Here's how the part is built. I have some questions about the finished solid (model axes, mm). Give positions to 0.01 mm unless a question says otherwise; leave off trailing zeros. Order: outer loops, then holes, each group sorted by start corner. A loop starts at its lowest first (then second) coordinate and runs counter-clockwise, first axis right, second up.
from build123d import *

# Parameters (mm, degrees)
SKETCH_1_W          = 61.702142611
SKETCH_1_H          = 61.347239899
EXTRUDE_1_DEPTH     = 2
SKETCH_2_W          = 9
SKETCH_2_H          = 6
CUT_EXTRUDE_1_DEPTH = 2


with BuildPart() as part:
    # 草图1 → 凸台-拉伸1 (new body)
    with BuildSketch(Plane(origin=(-129.641159043, -2421.788142989, -243.940490516), x_dir=(1, 0, 0), z_dir=(0, 1, 0))):
        with BuildLine():
            Line((-116.231072015, -154.924864972), (-44.528929404, -154.924864972))
            ThreePointArc((-44.528929404, -154.924864972), (-43.114715842, -155.510651409), (-42.528929404, -156.924864972))
            Line((-42.528929404, -156.924864972), (-42.528929404, -226.272104871))
            ThreePointArc((-42.528929404, -226.272104871), (-43.114715842, -227.686318433), (-44.528929404, -228.272104871))
            Line((-44.528929404, -228.272104871), (-116.231072015, -228.272104871))
            ThreePointArc((-116.231072015, -228.272104871), (-117.645285578, -227.686318433), (-118.231072015, -226.272104871))
            Line((-118.231072015, -226.272104871), (-118.231072015, -156.924864972))
            ThreePointArc((-118.231072015, -156.924864972), (-117.645285578, -155.510651409), (-116.231072015, -154.924864972))
        make_face()
        with Locations((-80.38000071, -191.598484922)):
            Rectangle(SKETCH_1_W, SKETCH_1_H, mode=Mode.SUBTRACT)
    extrude(amount=EXTRUDE_1_DEPTH)

    # 草图2 → 切除-拉伸1 (cut)
    with BuildSketch(Plane(origin=(0, -2419.788142989, 0), x_dir=(1, 0, 0), z_dir=(0, 1, 0))):
        with Locations((-232.033164197, 86.015625544)):
            Rectangle(SKETCH_2_W, SKETCH_2_H)
    extrude(amount=-CUT_EXTRUDE_1_DEPTH, mode=Mode.SUBTRACT)


solid = part.part
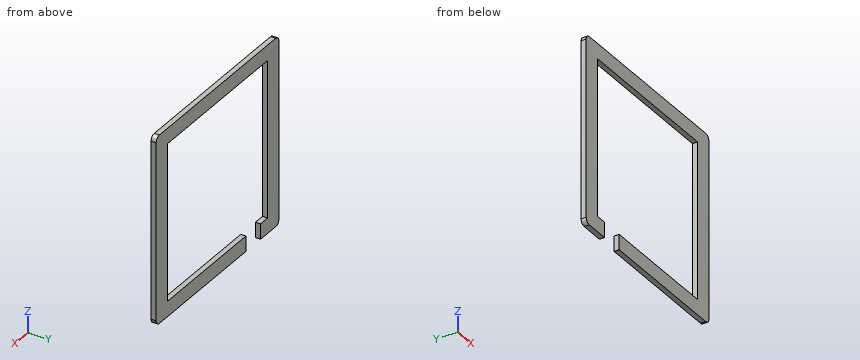
Q1. I'm going to push a flat-ended pin straight in: P1, Ø10, axis at x = -206, z = -80, coming from the +Y side. Where does the tip first touch, or does it pass through?
Filled sheet:
P1: stops at y = -2419.79
Q2. If we section it at C-C on y = -2421.25: List the corners of the cut face in (x, z) for me, plus the area to 3 significant figures.
Filled sheet:
outline: (-247.87, -87.02) arc R2 ccw to (-245.87, -89.02) - (-236.53, -89.02) - (-236.53, -83.02) - (-240.87, -83.02) - (-240.87, -21.67) - (-179.17, -21.67) - (-179.17, -83.02) - (-227.53, -83.02) - (-227.53, -89.02) - (-174.17, -89.02) arc R2 ccw to (-172.17, -87.02) - (-172.17, -17.67) arc R2 ccw to (-174.17, -15.67) - (-245.87, -15.67) arc R2 ccw to (-247.87, -17.67) - close
area: 1,710 mm2
Q3. I need wall thicknesses on L1, parallel to X at y = -2421.05, z = -73; L2, parallel to Z at x = -196.5, y = -2421.5; L3, parallel to Z at x = -236, y = -2420.5. Which ranges of each line are inside material? Lowest first, please.
Filled sheet:
L1: x = -247.87 to -240.87, -179.17 to -172.17
L2: z = -89.02 to -83.02, -21.67 to -15.67
L3: z = -21.67 to -15.67
Q4. If we section it at A-A on x = -189.5: List the corners of the cut face in (y, z) for me.
Filled sheet:
outline: (-2421.79, -89.02) - (-2419.79, -89.02) - (-2419.79, -83.02) - (-2421.79, -83.02) - close; (-2421.79, -21.67) - (-2419.79, -21.67) - (-2419.79, -15.67) - (-2421.79, -15.67) - close
Q5. If we section it at D-D on x = -229.5: List the corners of the cut face in (y, z) for me.
Filled sheet:
outline: (-2421.79, -21.67) - (-2419.79, -21.67) - (-2419.79, -15.67) - (-2421.79, -15.67) - close
Q6. If we section it at B-B on z = -80.5: List the corners of the cut face in (x, y) for me.
Filled sheet:
outline: (-247.87, -2421.79) - (-240.87, -2421.79) - (-240.87, -2419.79) - (-247.87, -2419.79) - close; (-179.17, -2421.79) - (-172.17, -2421.79) - (-172.17, -2419.79) - (-179.17, -2419.79) - close
